Input: part model. Units: mm. Frame: model coordinates. Coordinates: 2 decimals unless noted, no trailing zeros. Loops run counter-clockwise (first coordinate to the right, second up) from the corner with the lowest first, then second, coordinate; pieces in that order, holes last.
(1) Contact query for a flat-ended pin moving along its axis: P1, Ø4, axis at x = 25.4, z = -50.8, coming from the +Y side. Output: stop coordinate, or through.
(2) Section B-B, the plane z = 0. Return loops of the section in (x, y).
(3) Section A-A, the plane z = -50.8. Return loops of the section in (x, y).
(4) Section D-D, the plane y = 0.9. Give the number of separate pieces and of enclosed holes in the cut face, then the cut area to 3 significant figures.
(5) Section C-C, the plane x = 8. Return loops of the section in (y, z).
(6) Line query: L1, parallel to Z at x = 12.7, y = 0.3; L2, parallel to X at y = 0.8, z = -49.5; L3, parallel to Z at x = 17, y = 1.4. Output: solid intervals per line, ascending.
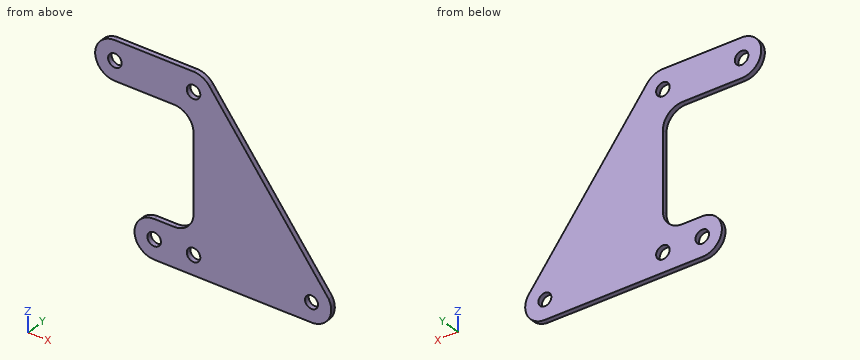
Autodesk Inventor part; units mm, degrees
ref_plane "YZ Plane" through (0, 0, 0) normal (1, 0, 0) x (0, 1, 0)
ref_plane "XZ Plane" through (0, 0, 0) normal (0, 1, 0) x (-1, 0, 0)
ref_plane "XY Plane" through (0, 0, 0) normal (0, 0, 1) x (1, 0, 0)
sketch "main" plane through (0, 0, 0) normal (0, 0, 1) x (1, 0, 0)
  circle A0 centre (33.5416, 32.0006) radius 2.1844
  line L0 (8.1416, 38.3506) -> (33.5416, 38.3506)
  line L1 (33.5416, 25.6506) -> (14.4916, 25.6506)
  arc A1 (33.5416, 25.6506) -> (33.5416, 38.3506) centre (33.5416, 32.0006) ccw
  circle A2 centre (8.1416, 32.0006) radius 2.1844
  arc A3 (14.4916, 25.6506) -> (8.1416, 19.3006) centre (14.4916, 19.3006) ccw
  arc A4 (8.1416, 38.3506) -> (2.462, 34.8404) centre (8.1416, 32.0006) ccw
  line L2 (8.1416, -6.0994) -> (8.1416, 19.3006)
  arc A5 (8.1416, -6.0994) -> (14.4916, -12.4494) centre (14.4916, -6.0994) ccw
  circle A6 centre (8.1416, -18.7994) radius 2.1844
  line L3 (14.4916, -12.4494) -> (20.8416, -12.4494)
  line L4 (-29.9584, -25.1494) -> (20.8416, -25.1494)
  arc A7 (20.8416, -25.1494) -> (20.8416, -12.4494) centre (20.8416, -18.7994) ccw
  circle A8 centre (20.8416, -18.7994) radius 2.1844
  circle A9 centre (-29.9584, -18.7994) radius 2.0955
  arc A10 (-34.5524, -14.4156) -> (-29.9584, -25.1494) centre (-29.9584, -18.7994) ccw
  line L5 (-35.4577, -15.6244) -> (3.0589, 35.807)
  point P0 (9.5067, 8.1196)
  point P1 (8.1416, 25.6506)
  point P2 (8.1416, -12.4494)
  dimension "d0" = 6.35
  dimension "d4" = 4.191
sketch "Sketch1" plane through (0, 0, 0) normal (0, 1, 0) x (-1, 0, 0)
  circle A0 centre (0, 0) radius 2.1844
  line L0 (-25.4, 6.35) -> (0, 6.35)
  line L1 (0, -6.35) -> (-19.05, -6.35)
  arc A1 (0, -6.35) -> (0, 6.35) centre (0, 0) ccw
  circle A2 centre (-25.4, 0) radius 2.1844
  arc A3 (-19.05, -6.35) -> (-25.4, -12.7) centre (-19.05, -12.7) ccw
  arc A4 (-25.4, 6.35) -> (-31.0796, 2.8398) centre (-25.4, 0) ccw
  line L2 (-25.4, -38.1) -> (-25.4, -12.7)
  arc A5 (-25.4, -38.1) -> (-19.05, -44.45) centre (-19.05, -38.1) ccw
  circle A6 centre (-25.4, -50.8) radius 2.1844
  line L3 (-19.05, -44.45) -> (-12.7, -44.45)
  line L4 (-63.5, -57.15) -> (-12.7, -57.15)
  arc A7 (-12.7, -57.15) -> (-12.7, -44.45) centre (-12.7, -50.8) ccw
  circle A8 centre (-12.7, -50.8) radius 2.1844
  circle A9 centre (-63.5, -50.8) radius 2.0955
  arc A10 (-68.094, -46.4162) -> (-63.5, -57.15) centre (-63.5, -50.8) ccw
  line L5 (-68.9993, -47.625) -> (-30.4827, 3.8064)
extrude "Extrusion1" add sketch "Sketch1" along normal blind 1.5875 contours L0 A1 L1 A3 L2 A5 L3 A7 L4 A10 L5 A4
properties part number "gusset" material "Acetal Resin, White"
Report:
1. P1: passes through
2. outline: (-6.35, 0) - (-2.18, 0) - (-2.18, 1.59) - (-6.35, 1.59) - close; (2.18, 0) - (23.22, 0) - (23.22, 1.59) - (2.18, 1.59) - close; (27.58, 0) - (33.33, 0) - (33.33, 1.59) - (27.58, 1.59) - close
3. outline: (6.35, 0) - (10.52, 0) - (10.52, 1.59) - (6.35, 1.59) - close; (14.88, 0) - (23.22, 0) - (23.22, 1.59) - (14.88, 1.59) - close; (27.58, 0) - (61.4, 0) - (61.4, 1.59) - (27.58, 1.59) - close; (65.6, 0) - (69.85, 0) - (69.85, 1.59) - (65.6, 1.59) - close
4. separate pieces: 1
4. enclosed holes: 5
4. area: 2,230 mm2
5. outline: (0, -55.07) - (1.59, -55.07) - (1.59, -46.53) - (0, -46.53) - close; (0, -6.35) - (1.59, -6.35) - (1.59, 6.35) - (0, 6.35) - close
6. L1: z = -57.15 to -52.98, -48.62 to -44.45, -6.35 to 6.35
6. L2: x = 6.48 to 10.94, 14.46 to 23.64, 27.16 to 61.86, 65.14 to 69.72
6. L3: z = -57.15 to -44.45, -6.35 to 6.35
